Input: part model. Units: mm. Frame: model coordinates. Face numbers are marked on the shaded views. A direction names the side the tool comes from. Give positions to 0.01 mm unless a question says otherwise; leave off trailing zeros. Loops run counter-clockwise (first coordinate to the right, second up) from the corner with the lowest first, then second, coordinate; pieces in that order, holes last.
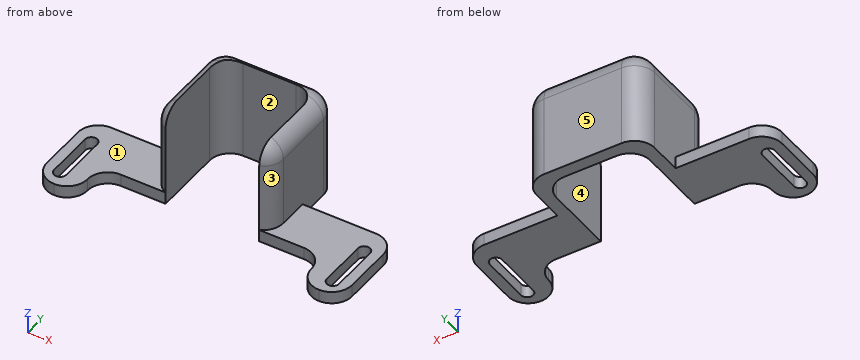
from build123d import *

# Parameters (mm, degrees)
F2_DEPTH     = 25
F3_DEPTH     = 3
F4_DEPTH     = 25
F5_R         = 4.99999
F6_T1_DEPTH  = 25
F6_T3_DEPTH  = 25
F6_T5_DEPTH  = 50
F6_T7_DEPTH  = 33.4564392374
F6_T9_DEPTH  = 50
F6_T11_DEPTH = 33.4564392374
F7_T1_DEPTH  = 15.417424305
F7_T3_DEPTH  = 19
F7_T6_ANGLE  = 89.9999999974
F7_T8_ANGLE  = 89.9999999974
F7_T10_ANGLE = 209.6926070845
F7_T12_ANGLE = 209.6926070845


# Not quite as in the source:
# - a fillet or chamfer that OpenCascade refuses, or shapes differently, is made with other operations: its cross-section is extruded or revolved along the edge and cut away or added
# - a fillet or chamfer is up to 0.001 mm smaller than in the source, because OpenCascade refuses the exact size


with BuildPart() as f2:
    # F0 (on Top) → F2 (new body)
    with BuildSketch(Plane.XY):
        Polygon((14.5, 35), (0, 35), (-14.5, 35), (-14.5, 22), (-14.5, 10), (-11.5, 10), (-11.5, 32), (0, 32), (11.5, 32), (11.5, 10), (14.5, 10), (14.5, 22), align=None)
    extrude(amount=F2_DEPTH)

    # F0 (on Top) → F3 (join)
    with BuildSketch(Plane.XY):
        Polygon((-14.5, 10), (-14.5, 22), (-37.5, 22), (-37.5, 0), (-27.5, 0), (-27.5, 10), align=None)
        Polygon((37.5, 22), (14.5, 22), (14.5, 10), (27.5, 10), (27.5, 0), (37.5, 0), align=None)
    extrude(amount=F3_DEPTH)

    # F1 (on Top) → F4 (cut)
    with BuildSketch(Plane.XY):
        with BuildLine():
            Line((35, 3.8767794613), (35, 15.8767794613))
            ThreePointArc((35, 15.8767794613), (33.5, 17.3767794613), (32, 15.8767794613))
            Line((32, 15.8767794613), (32, 3.8767794613))
            ThreePointArc((32, 3.8767794613), (33.5, 2.3767794613), (35, 3.8767794613))
        make_face()
        with BuildLine():
            ThreePointArc((-32, 15.8767794613), (-33.5, 17.3767794613), (-35, 15.8767794613))
            Line((-35, 15.8767794613), (-35, 3.8767794613))
            ThreePointArc((-35, 3.8767794613), (-33.5, 2.3767794613), (-32, 3.8767794613))
            Line((-32, 3.8767794613), (-32, 15.8767794613))
        make_face()
    extrude(amount=F4_DEPTH, mode=Mode.SUBTRACT)

    # F5 (radius 5 in the source; OpenCascade refuses exactly that, so slightly less here)
    f5_edges = [f2.edges().sort_by_distance(p)[0] for p in [
        (-37.5, 0, 1.5),
        (-27.5, 0, 1.5),
        (-37.5, 22, 1.5),
        (37.5, 22, 1.5),
        (37.5, 0, 1.5),
        (27.5, 0, 1.5),
        (27.5, 10, 1.5),
        (-27.5, 10, 1.5),
    ]]
    fillet(f5_edges, radius=F5_R)

    # F6: fillet of radius 5 on 6 edges, made by hand

    # F6_s2 → F6_t1 (join)
    with BuildSketch(Plane.XY):
        with BuildLine():
            ThreePointArc((11.5, 27), (10.0355339059, 30.5355339059), (6.5, 32))
            Line((6.5, 32), (11.5, 32))
            Line((11.5, 32), (11.5, 27))
        make_face()
    extrude(amount=F6_T1_DEPTH)

    # F6_s4 → F6_t3 (join)
    with BuildSketch(Plane.XY):
        with BuildLine():
            ThreePointArc((-6.5, 32), (-10.0355339059, 30.5355339059), (-11.5, 27))
            Line((-11.5, 27), (-11.5, 32))
            Line((-11.5, 32), (-6.5, 32))
        make_face()
    extrude(amount=F6_T3_DEPTH)

    # F6_s6 → F6_t5 (cut)
    with BuildSketch(Plane.XY.offset(-12.5)):
        with BuildLine():
            ThreePointArc((14.5, 30), (13.0355339059, 33.5355339059), (9.5, 35))
            Line((9.5, 35), (14.5, 35))
            Line((14.5, 35), (14.5, 30))
        make_face()
    extrude(amount=F6_T5_DEPTH, mode=Mode.SUBTRACT)

    # F6_s8 → F6_t7 (cut)
    with BuildSketch(Plane.XY.offset(3)):
        with BuildLine():
            ThreePointArc((11.5, 10), (13.6833001327, 11.8439629074), (14.5, 14.582575695))
            Line((14.5, 14.582575695), (14.5, 10))
            Line((14.5, 10), (11.5, 10))
        make_face()
    extrude(amount=F6_T7_DEPTH, mode=Mode.SUBTRACT)

    # F6_s10 → F6_t9 (cut)
    with BuildSketch(Plane.XY.offset(-12.5)):
        with BuildLine():
            ThreePointArc((-9.5, 35), (-13.0355339059, 33.5355339059), (-14.5, 30))
            Line((-14.5, 30), (-14.5, 35))
            Line((-14.5, 35), (-9.5, 35))
        make_face()
    extrude(amount=F6_T9_DEPTH, mode=Mode.SUBTRACT)

    # F6_s12 → F6_t11 (cut)
    with BuildSketch(Plane.XY.offset(3)):
        with BuildLine():
            ThreePointArc((-11.5, 10), (-13.6833001327, 11.8439629074), (-14.5, 14.582575695))
            Line((-14.5, 14.582575695), (-14.5, 10))
            Line((-14.5, 10), (-11.5, 10))
        make_face()
    extrude(amount=F6_T11_DEPTH, mode=Mode.SUBTRACT)

    # F7: fillet of radius 5 on 3 edges, made by hand

    # F7_s2 → F7_t1 (cut)
    with BuildSketch(Plane.XZ.offset(-30)):
        with BuildLine():
            ThreePointArc((-9.5, 25), (-13.0355339059, 23.5355339059), (-14.5, 20))
            Line((-14.5, 20), (-14.5, 25))
            Line((-14.5, 25), (-9.5, 25))
        make_face()
        with BuildLine():
            ThreePointArc((9.5, 25), (13.0355339059, 23.5355339059), (14.5, 20))
            Line((14.5, 20), (14.5, 25))
            Line((14.5, 25), (9.5, 25))
        make_face()
    extrude(amount=F7_T1_DEPTH, mode=Mode.SUBTRACT)

    # F7_s4 → F7_t3 (cut)
    with BuildSketch(Plane.YZ.offset(-9.5)):
        with BuildLine():
            ThreePointArc((30, 25), (33.5355339059, 23.5355339059), (35, 20))
            Line((35, 20), (35, 25))
            Line((35, 25), (30, 25))
        make_face()
    extrude(amount=F7_T3_DEPTH, mode=Mode.SUBTRACT)

    # F7_s5 → F7_t6 (revolve, cut)
    with BuildSketch(Plane.YZ.offset(9.4999999999)):
        with BuildLine():
            ThreePointArc((30, 25), (33.5355339059, 23.5355339059), (35, 20))
            Line((35, 20), (35, 25))
            Line((35, 25), (30, 25))
        make_face()
    revolve(axis=Axis((9.4999999999, 29.9999999999, 25), (0, 0, -1)), revolution_arc=F7_T6_ANGLE, mode=Mode.SUBTRACT)

    # F7_s7 → F7_t8 (revolve, cut)
    with BuildSketch(Plane.XZ.offset(-29.9999999999)):
        with BuildLine():
            ThreePointArc((-9.5, 25), (-13.0355339059, 23.5355339059), (-14.5, 20))
            Line((-14.5, 20), (-14.5, 25))
            Line((-14.5, 25), (-9.5, 25))
        make_face()
    revolve(axis=Axis((-9.4999999999, 29.9999999999, 25), (0, 0, -1)), revolution_arc=F7_T8_ANGLE, mode=Mode.SUBTRACT)

    # F7_s9 → F7_t10 (revolve, cut)
    with BuildSketch(Plane.XZ.offset(-14.5825756948)):
        with BuildLine():
            ThreePointArc((14.5, 20), (13.0355339059, 23.5355339059), (9.5, 25))
            Line((9.5, 25), (14.5, 25))
            Line((14.5, 25), (14.5, 20))
        make_face()
    revolve(axis=Axis((9.5000000002, 14.5825756948, 25), (0, 0, -1)), revolution_arc=F7_T10_ANGLE, mode=Mode.SUBTRACT)

    # F7_s11 → F7_t12 (revolve, cut)
    with BuildSketch(Plane(origin=(-8.6059581245, 15.0923752984, 0), x_dir=(0, 0, 1), z_dir=(-0.4953465841, 0.8686954366, 0))):
        with BuildLine():
            ThreePointArc((25, -1.02917759), (23.5355339059, 2.506356316), (20, 3.97082241))
            Line((20, 3.97082241), (25, 3.97082241))
            Line((25, 3.97082241), (25, -1.02917759))
        make_face()
    revolve(axis=Axis((-9.5000000002, 14.5825756948, 25), (0, 0, -1)), revolution_arc=F7_T12_ANGLE, mode=Mode.SUBTRACT)


solid = f2.part
(1) Pin query (flat end, axial travel): pin 1 Ø1.5 at (x, z) = (15, 1.5) entering from -Y; pin 2 Ø4 at (y, z) = (25, 8) entering from +X; pin 3 Ø1 at (y, z) = (25.5, 22) entering from +X. Return the tip coordinate at first contact, or that it passes through.
Values follow:
pin 1: stops at y = 10
pin 2: stops at x = 14.5
pin 3: stops at x = 14.27
(2) Ray query, probe 1 along X at (y, z) = (21, 8.75); probe 2 along Z at (x, y) = (-29, 21); probe 3 along X at (y, z) = (29.5, 7). Return the intervals inside material, ascending.
Values follow:
probe 1: x = -14.5 to -11.5, 11.5 to 14.5
probe 2: z = 0 to 3
probe 3: x = -14.5 to -10.83, 10.83 to 14.5
(3) Cut plane B-B (z = 18). Return the cut outline in (x, y).
Values follow:
outline: (-14.5, 14.58) arc R5 ccw to (-11.5, 10) - (-11.5, 27) arc R5 cw to (-6.5, 32) - (6.5, 32) arc R5 cw to (11.5, 27) - (11.5, 10) arc R5 ccw to (14.5, 14.58) - (14.5, 30) arc R5 ccw to (9.5, 35) - (-9.5, 35) arc R5 ccw to (-14.5, 30) - close
(4) Reachability of the marked faces 4 and 5 from +Z, -Z, +X, -X, +Y, -Y: full face, straight path, thin tool, end or side. Return the list, or none.
Values follow:
face 4: +Z, -Z, -Y
face 5: +Z, -Z, +X, -X, +Y
(5) Cut plane A-A (y = 29). Return the cut outline in (x, z).
Values follow:
outline: (-14.5, 0) - (-11.08, 0) - (-11.08, 24.74) arc R5 ccw to (-14.5, 20) - close; (11.08, 0) - (14.5, 0) - (14.5, 20) arc R5 ccw to (11.08, 24.74) - close
(6) Cut plane D-D (y = 7). Return the cut outline in (x, z), and give its area (3 significant figures).
Values follow:
outline: (-37.5, 0) - (-35, 0) - (-35, 3) - (-37.5, 3) - close; (-32, 0) - (-27.08, 0) - (-27.08, 3) - (-32, 3) - close; (27.08, 0) - (32, 0) - (32, 3) - (27.08, 3) - close; (35, 0) - (37.5, 0) - (37.5, 3) - (35, 3) - close
area: 44.5 mm2
(7) Mould query, pull axis X, two halves, no side actions, for the marked faces 1, 2 and 3. Classes: +X half, -X half, draft (parallel to the pull), parting line (faces both ways), or undercut.
Values follow:
face 1: draft
face 2: undercut
face 3: +X half
(8) Cut plane C-C (x = 33.5). Return the cut outline in (y, z).
Values follow:
outline: (0.1, 0) - (2.38, 0) - (2.38, 3) - (0.1, 3) - close; (17.38, 0) - (21.9, 0) - (21.9, 3) - (17.38, 3) - close
